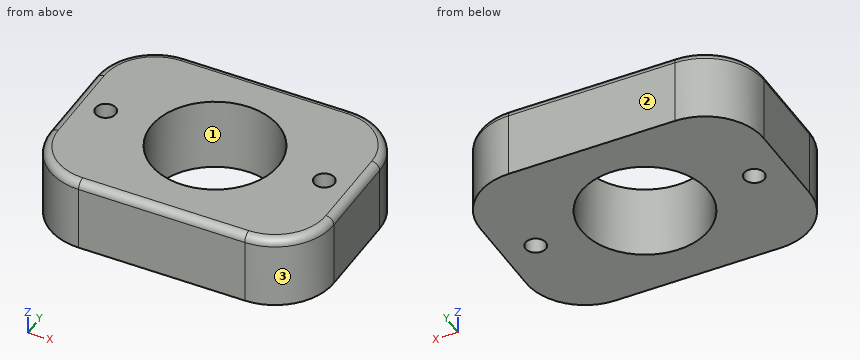
from build123d import *

# Parameters (mm, degrees)
F0_R     = 2.286
F0_R_2   = 14.2875
F1_DEPTH = 16.51
F2_R     = 1.778


with BuildPart() as f1:
    # F0 (on Top) → F1 (new body)
    with BuildSketch(Plane.XY):
        with BuildLine():
            Line((-18.70075, -23.1775), (18.70075, -23.1775))
            ThreePointArc((18.70075, -23.1775), (28.0402163659, -19.3089663659), (31.90875, -9.9695))
            Line((31.90875, -9.9695), (31.90875, 9.9695))
            ThreePointArc((31.90875, 9.9695), (28.0402163659, 19.3089663659), (18.70075, 23.1775))
            Line((18.70075, 23.1775), (-18.70075, 23.1775))
            ThreePointArc((-18.70075, 23.1775), (-28.0402163659, 19.3089663659), (-31.90875, 9.9695))
            Line((-31.90875, 9.9695), (-31.90875, -9.9695))
            ThreePointArc((-31.90875, -9.9695), (-28.0402163659, -19.3089663659), (-18.70075, -23.1775))
        make_face()
        with BuildLine():
            Line((-18.70075, 20.6375), (18.70075, 20.6375))
            ThreePointArc((18.70075, 20.6375), (26.2441651417, 17.5129151417), (29.36875, 9.9695))
            Line((29.36875, 9.9695), (29.36875, -9.9695))
            ThreePointArc((29.36875, -9.9695), (26.2441651417, -17.5129151417), (18.70075, -20.6375))
            Line((18.70075, -20.6375), (-18.70075, -20.6375))
            ThreePointArc((-18.70075, -20.6375), (-26.2441651417, -17.5129151417), (-29.36875, -9.9695))
            Line((-29.36875, -9.9695), (-29.36875, 9.9695))
            ThreePointArc((-29.36875, 9.9695), (-26.2441651417, 17.5129151417), (-18.70075, 20.6375))
        make_face(mode=Mode.SUBTRACT)
        with BuildLine():
            ThreePointArc((29.36875, 9.9695), (26.2441651417, 17.5129151417), (18.70075, 20.6375))
            Line((18.70075, 20.6375), (-18.70075, 20.6375))
            ThreePointArc((-18.70075, 20.6375), (-26.2441651417, 17.5129151417), (-29.36875, 9.9695))
            Line((-29.36875, 9.9695), (-29.36875, -9.9695))
            ThreePointArc((-29.36875, -9.9695), (-26.2441651417, -17.5129151417), (-18.70075, -20.6375))
            Line((-18.70075, -20.6375), (18.70075, -20.6375))
            ThreePointArc((18.70075, -20.6375), (26.2441651417, -17.5129151417), (29.36875, -9.9695))
            Line((29.36875, -9.9695), (29.36875, 9.9695))
        make_face()
        with Locations((-24.60625, 0)):
            Circle(F0_R, mode=Mode.SUBTRACT)
        Circle(F0_R_2, mode=Mode.SUBTRACT)
        with Locations((24.60625, 0)):
            Circle(F0_R, mode=Mode.SUBTRACT)
    extrude(amount=F1_DEPTH)

    # F2
    f2_edges = [f1.edges().sort_by_distance(p)[0] for p in [
        (28.040216, 19.308966, 16.51),
    ]]
    fillet(f2_edges, radius=F2_R)


solid = f1.part
Could you check a few things on this model? Use its own coordinates, in mm. Face numbers are marked on the shaded views. Give positions to 0.01 mm unless a question says otherwise; leave off trailing zeros. Order: outer loops, then holes, each group sorted by start corner. A loop starts at its lowest first (then second) coordinate and runs counter-clockwise, first axis right, second up. Notation, with made-up numbers: (40, 20) -> (50, 20) arc R23 cw to (50, 49) -> close; hole circle Ø6 at (-9.75, 71.5). An arc over 180 degrees is marked (long way). Return JSON: item names as keys, results as strings.
1. Imagine slicing it at B-B on y = 0. List the corners of the cut face in (x, z) for me.
Answer list:
{"outline": "(-31.91, 0) -> (-26.89, 0) -> (-26.89, 16.51) -> (-30.13, 16.51) arc R1.78 ccw to (-31.91, 14.73) -> close; (-22.32, 0) -> (-14.29, 0) -> (-14.29, 16.51) -> (-22.32, 16.51) -> close; (14.29, 0) -> (22.32, 0) -> (22.32, 16.51) -> (14.29, 16.51) -> close; (26.89, 0) -> (31.91, 0) -> (31.91, 14.73) arc R1.78 ccw to (30.13, 16.51) -> (26.89, 16.51) -> close"}
2. I need wall thicknesses on line 1 (Y direction, x = 0, z = 6.75); line 2 (Y direction, x = 26.5, z = 2); line 3 (X direction, y = -3.5, z = 1.75). Which ranges of each line are inside material? Lowest first, please. Write a range as from..to.
Answer list:
{"line 1": "y = -23.18..-14.29, 14.29..23.18", "line 2": "y = -20.63..-1.28, 1.28..20.63", "line 3": "x = -31.91..-13.85, 13.85..31.91"}
3. For pin 1 Ø5.5 at (x, y) = (24.61, 0) entering from -Z; pin 2 Ø1.5 at (y, z) = (-17.5, 12) entering from -X; pin 3 Ø3 at (y, z) = (-15.5, 4) entering from +X, each with a flat end and sliding along its axis, tell me the tip position at first contact or that it passes through.
Answer list:
{"pin 1": "stops at z = 0", "pin 2": "stops at x = -30.04", "pin 3": "stops at x = 31.28"}
4. Imagine slicing it at C-C on z = 7.5. List the corners of the cut face in (x, y) for me (1 decimal), then the cut area to 3 significant figures.
Answer list:
{"outline": "(-31.9, -10) arc R13.2 ccw to (-18.7, -23.2) -> (18.7, -23.2) arc R13.2 ccw to (31.9, -10) -> (31.9, 10) arc R13.2 ccw to (18.7, 23.2) -> (-18.7, 23.2) arc R13.2 ccw to (-31.9, 10) -> close; hole circle Ø4.6 at (-24.6, 0); hole circle Ø28.6 at (0, 0); hole circle Ø4.6 at (24.6, 0)", "area": "2,130 mm2"}
5. Thinking about a two-plate mould opening in Y: for the marked faces 1, 2 and 3, which applies, pulls with the +Y half, pulls with the -Y half, needs draft (parallel to the pull), parting line crosses it, or undercut?
Answer list:
{"face 1": "undercut", "face 2": "pulls with the +Y half", "face 3": "pulls with the -Y half"}
6. Imagine slicing it at A-A on x = 0. List the corners of the cut face in (y, z) for me, then the cut area to 3 significant figures.
Answer list:
{"outline": "(-23.18, 0) -> (-14.29, 0) -> (-14.29, 16.51) -> (-21.4, 16.51) arc R1.78 ccw to (-23.18, 14.73) -> close; (14.29, 0) -> (23.18, 0) -> (23.18, 14.73) arc R1.78 ccw to (21.4, 16.51) -> (14.29, 16.51) -> close", "area": "292 mm2"}
